The listing builds one solid part. Answer for the finished solid, in the listing's coordinates (mm). Face numbers are marked on the shaded views. Round coordinates to 2 decimals unless told otherwise and drop trailing zeros. Order: outer loops, then holes, each group sorted by start corner. A loop starts at its lowest first (then second) coordinate and runs counter-clockwise, first axis right, second up. Notation, with made-up numbers: M -15,3.5 L 11,3.5 A28 ccw 11,38.5 Z; hole C -11.5,50 d3. An arc over 180 degrees is marked long. Write item = value, one per line. Start each with the question number.
(1) Straight lines are drawn through the part: probe 1 along Y at (x, z) = (1.6, 0); probe 2 along Z at (x, y) = (3.15, 16); probe 3 along Y at (x, z) = (0.55, -4). For each, find the intervals that lie inside material, in ascending order. Write a range as from..to.
(2) For a pull along Y with two mould halves and no side action, classify the marked faces 1, 2 and 3 as released by +Y, released by -Y, zero draft, split by the parting line, or undercut.
(3) A cutting plane is placed at A-A, the plane y = 45.5. Determine the outline of the cut face in (x, z), and give its area (3 significant figures).
(4) Each of these flat-tipped pins is pushed along its axis until it touches: pin 1 (1 mm diameter, centred on x = 4, z = 4.5, fed in from +Y); pin 2 (1.5 mm diameter, centred on x = 4, y = 25.5, fed in from +Z); pin 3 (3.5 mm diameter, centred on y = 0, z = 0, fed in from +X). Where does it stop, or does it pass through?
from build123d import *

# Parameters (mm, degrees)
BASPROSKE_W        = 5
BASPROSKE_H        = 18
TOOTHCUT_DEPTH     = 26.942243542
TEETHCUTS_COUNT    = 30
BORSKE_R           = 3
BORE_DEPTH         = 50.0000508
BOSS_EXTRU_1_DEPTH = 5


with BuildPart() as part:
    # BasProSke → Base-Revolve (revolve)
    with BuildSketch(Plane(origin=(0, 0, 0), x_dir=(1, 0, 0), z_dir=(0, 1, 0)), mode=Mode.PRIVATE) as base_revolve_sk:
        with Locations((2.5, 9)):
            Rectangle(BASPROSKE_W, BASPROSKE_H)
    revolve(base_revolve_sk.sketch.rotate(Axis((-10, 0, 0), (1, 0, 0)), 180), axis=Axis((-10, 0, 0), (1, 0, 0)))

    # TooCutSke → ToothCut (cut, through all)
    with BuildSketch(Plane(origin=(0, 0, 0), x_dir=(0, 0, -1), z_dir=(1, 0, 0))):
        with BuildLine():
            ThreePointArc((0.523521522, 15.458887906), (0, 15.46775), (-0.523521522, 15.458887906))
            ThreePointArc((-0.523521522, 15.458887906), (-0.919551256, 16.760900189), (-1.568701479, 17.957010353))
            ThreePointArc((-1.568701479, 17.957010353), (0, 18.0254), (1.568701479, 17.957010353))
            ThreePointArc((1.568701479, 17.957010353), (0.919551256, 16.760900189), (0.523521522, 15.458887906))
        make_face()
    toothcut = extrude(amount=TOOTHCUT_DEPTH, mode=Mode.SUBTRACT)

    # TeethCuts: ToothCut ×30 about axis
    teethcuts_axis = Axis((0, 0, 0), (1, 0, 0))
    for i in range(1, TEETHCUTS_COUNT):
        add(toothcut.rotate(teethcuts_axis, i * 360 / TEETHCUTS_COUNT), mode=Mode.SUBTRACT)

    # BorSke → Bore (cut, symmetric)
    with BuildSketch(Plane(origin=(0, 0, 0), x_dir=(0, 0, -1), z_dir=(1, 0, 0))):
        with Locations(Location((0, 0, 0), (0, 0, 180))):
            Circle(BORSKE_R)
    extrude(amount=BORE_DEPTH, both=True, mode=Mode.SUBTRACT)

    # Esquisse2 → Boss.-Extru.1 (add)
    with BuildSketch(Plane(origin=(5, 0, 0), x_dir=(0, 0, -1), z_dir=(1, 0, 0))):
        Polygon((-3.726164843, 15.01222787), (-11.656542396, 50.01222787), (7.45003198, 67.64568515), (-0.54996802, 69.468919999), (-18.921674151, 52.513672615), (-9.091715336, 12.513672615), align=None)
    extrude(amount=-BOSS_EXTRU_1_DEPTH)


solid = part.part
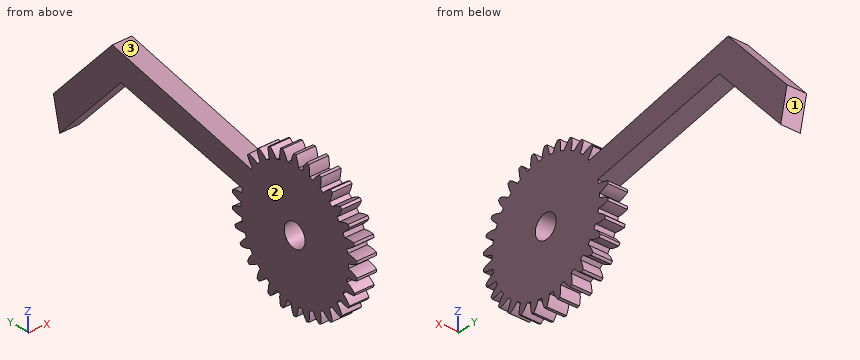
Reported:
q1.probe_1 = -15.47..-3, 3..15.47, 60.77..69.34
q1.probe_2 = -5.98..-4.25, -2.67..-0.65, 0.65..2.67, 3.95..9.95
q1.probe_3 = -15.58..15.58, 64.46..68.43
q2.face_1 = released by +Y
q2.face_2 = zero draft
q2.face_3 = undercut
q3.outline = M 0,10.63 L 5,10.63 L 5,17.2 L 0,17.2 Z
q3.area = 32.8 mm²
q4.pin_1 = 66.28
q4.pin_2 = 12.47
q4.pin_3 = through
